The model under review builds one solid part; all positions refer to its coordinate system, in mm. Face numbers are marked on the shaded views. A direction names the side the tool comes from. Round coordinates to 2 decimals unless told otherwise and drop trailing zeros. Order: outer loops, then holes, each group sorted by start corner. A loop starts at its lowest first (then second) coordinate and runs counter-clockwise, first axis right, second up.
1) Consider section A-A (z = -15). Give the boundary of the cut face in (x, y), then the cut area to 3 significant figures.
2) Consider section D-D (x = 42). Give the boundary of the cut face in (y, z), then the cut area to 3 significant figures.
3) Consider section C-C (y = 11.5). Give the boundary of the cut face in (x, z).
4) Mouldability with a two-part tool opening along Z and no side actions: class the marked faces 1, 2 and 3 as pulls with the +Z half, pulls with the -Z half, needs draft (parallel to the pull), parting line crosses it, or undercut.
5) Machinability: for the marked faces 4 and 5, which of the approach directions +Z, -Z, +X, -X, +Y, -Y give a long, thin tool a straight path to every point of the face, cutting with its end or side? Answer none if there is none.
6) Consider section B-B (x = 50). Give the boundary of the cut face in (y, z), then the cut area to 3 significant figures.
7) To check wall thickness, follow L1, parallel to X at y = 0.8, z = -15; L2, parallel to Z at x = 31, y = 6; L3, parallel to Y at x = 10, z = -27.95. State the ranges of each line that lie inside material, in increasing order.
8) Clearance check with flat-ended pins moving along their axes: P1, Ø5, axis at x = 39.5, z = -8, coming from the -Y side; P2, Ø3.5, axis at x = 10, z = -15, coming from the +Y side; P3, Ø3.5, axis at y = 8.5, z = -21, coming from the +X side; P4, Ø8, axis at y = 14, z = -7, coming from the -X side. State where each tip first meets the part, or that it passes through.
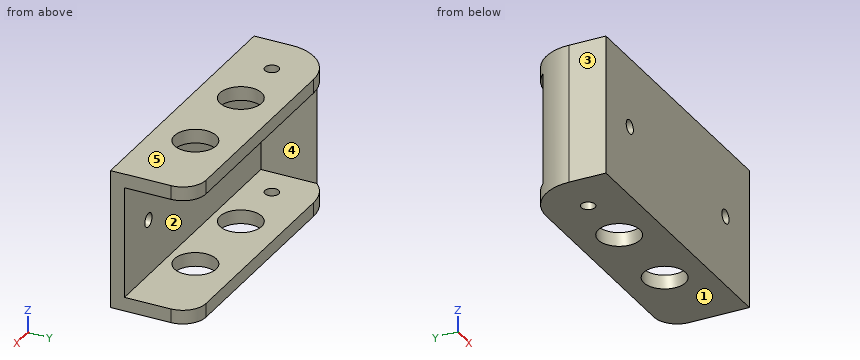
from build123d import *

# Parameters (mm, degrees)
CROQUIS1_W              = 60
CROQUIS1_H              = 30
CROQUIS1_R              = 1.5
SALIENTE_EXTRUIR1_DEPTH = 3
SALIENTE_EXTRUIR2_DEPTH = 15
REDONDEO1_R             = 10
REDONDEO2_R             = 5
CROQUIS3_R              = 4.5
CROQUIS3_R_2            = 1.5
CORTAR_EXTRUIR1_DEPTH   = 36


with BuildPart() as part:
    # Croquis1 → Saliente-Extruir1 (new body)
    with BuildSketch(Plane(origin=(0, 0, 0), x_dir=(1, 0, 0), z_dir=(0, 1, 0))):
        with Locations((30, 15)):
            Rectangle(CROQUIS1_W, CROQUIS1_H)
        with Locations(Location((10, 15, 0), (0, 0, 270))):
            Circle(CROQUIS1_R, mode=Mode.SUBTRACT)
        with Locations(Location((50, 15, 0), (0, 0, 270))):
            Circle(CROQUIS1_R, mode=Mode.SUBTRACT)
    extrude(amount=SALIENTE_EXTRUIR1_DEPTH)

    # Croquis2 → Saliente-Extruir2 (add)
    with BuildSketch(Plane(origin=(0, 3, 0), x_dir=(1, 0, 0), z_dir=(0, 1, 0))):
        Polygon((0, 30), (60, 30), (60, 27), (3, 27), (3, 3), (60, 3), (60, 0), (0, 0), align=None)
    extrude(amount=SALIENTE_EXTRUIR2_DEPTH)

    # Redondeo1
    # the kernel refuses this fillet: 10 mm, written as the material it takes off along each edge
    with BuildSketch(Plane(origin=(0, 18, 25), x_dir=(1, 0, 0), z_dir=(0, 0, -1))) as redondeo1_piece_1:
        with BuildLine():
            CenterArc((REDONDEO1_R, REDONDEO1_R), REDONDEO1_R, 180, 90)
            Line((0, REDONDEO1_R), (0, 0))
            Line((0, 0), (REDONDEO1_R, 0))
        make_face()
    extrude(amount=80, mode=Mode.SUBTRACT)

    # Redondeo2
    redondeo2_edges = [part.edges().sort_by_distance(p)[0] for p in [
        (60, 18, -1.5),
        (60, 18, -28.5),
    ]]
    fillet(redondeo2_edges, radius=REDONDEO2_R)

    # Croquis3 → Cortar-Extruir1 (cut)
    with BuildSketch(Plane.XY):
        with Locations((42, 9)):
            Circle(CROQUIS3_R)
        with Locations((23, 9)):
            Circle(CROQUIS3_R)
        with Locations((10, 9)):
            Circle(CROQUIS3_R_2)
    extrude(amount=-CORTAR_EXTRUIR1_DEPTH, mode=Mode.SUBTRACT)


solid = part.part
Answer below:
1. outline: (0, 0) - (8.5, 0) - (8.5, 3) - (3, 3) - (3, 15.14) arc R10 ccw to (0, 8) - close; (11.5, 0) - (48.5, 0) - (48.5, 3) - (11.5, 3) - close; (51.5, 0) - (60, 0) - (60, 3) - (51.5, 3) - close
1. area: 192 mm2
2. outline: (0, -30) - (4.5, -30) - (4.5, -27) - (3, -27) - (3, -3) - (4.5, -3) - (4.5, 0) - (0, 0) - close; (13.5, -30) - (18, -30) - (18, -27) - (13.5, -27) - close; (13.5, -3) - (18, -3) - (18, 0) - (13.5, 0) - close
2. area: 126 mm2
3. outline: (0.63, -30) - (19.26, -30) - (19.26, -27) - (3, -27) - (3, -3) - (19.26, -3) - (19.26, 0) - (0.63, 0) - close; (26.74, -30) - (38.26, -30) - (38.26, -27) - (26.74, -27) - close; (26.74, -3) - (38.26, -3) - (38.26, 0) - (26.74, 0) - close; (45.74, -30) - (60, -30) - (60, -27) - (45.74, -27) - close; (45.74, -3) - (60, -3) - (60, 0) - (45.74, 0) - close
4. face 1: pulls with the -Z half
4. face 2: undercut
4. face 3: needs draft
5. face 4: +X, +Y
5. face 5: +Z, +X, -X, +Y, -Y
6. outline: (0, -30) - (18, -30) - (18, -27) - (3, -27) - (3, -16.5) - (0, -16.5) - close; (0, -13.5) - (3, -13.5) - (3, -3) - (18, -3) - (18, 0) - (0, 0) - close
6. area: 171 mm2
7. L1: x = 0 to 8.5, 11.5 to 48.5, 51.5 to 60
7. L2: z = -30 to -27, -3 to 0
7. L3: y = 0 to 7.5, 10.5 to 18
8. P1: stops at y = 0
8. P2: stops at y = 3
8. P3: stops at x = 3
8. P4: stops at x = 0.2
